from build123d import *

# Parameters (mm, degrees)
BOSS_EXTRUDE1_DEPTH = 50.8
FILLET1_R           = 2.032
FILLET2_R           = 1.27
SKETCH2_R           = 2.1971
SKETCH2_R_2         = 15.875
CUT_EXTRUDE1_DEPTH  = 104.011248837
SKETCH3_W           = 1.47561847
SKETCH3_H           = 5.061923893
CUT_EXTRUDE2_DEPTH  = 0.635


with BuildPart() as part:
    # Sketch1 → Boss-Extrude1 (new body)
    with BuildSketch(Plane.XY):
        Polygon((85.725, 0), (-85.725, 0), (-87.558087105, -3.175), (-54.56251922, -22.225), (-52.3875, -22.225), (-52.3875, -6.35), (52.3875, -6.35), (52.3875, -22.225), (54.56251922, -22.225), (87.558087105, -3.175), align=None)
    extrude(amount=BOSS_EXTRUDE1_DEPTH)

    # Fillet1
    fillet1_edges = [part.edges().sort_by_distance(p)[0] for p in [
        (-85.725, 0, 25.4),
        (85.725, 0, 25.4),
        (87.558087105, -3.175, 25.4),
        (52.3875, -6.35, 25.4),
        (-52.3875, -6.35, 25.4),
        (-87.558087105, -3.175, 25.4),
    ]]
    fillet(fillet1_edges, radius=FILLET1_R)

    # Fillet2
    fillet2_edges = [part.edges().sort_by_distance(p)[0] for p in [
        (54.56251922, -22.225, 25.4),
        (52.3875, -22.225, 25.4),
        (-52.3875, -22.225, 25.4),
        (-54.56251922, -22.225, 25.4),
    ]]
    fillet(fillet2_edges, radius=FILLET2_R)

    # Sketch2 → Cut-Extrude1 (cut, through all)
    with BuildSketch(Plane(origin=(0, 0, 0), x_dir=(1, 0, 0), z_dir=(0, 1, 0))):
        with Locations(Location((6.35, -35.56, 0), (0, 0, 180))):
            Circle(SKETCH2_R)
        with Locations(Location((-6.35, -35.56, 0), (0, 0, 180))):
            Circle(SKETCH2_R)
        with Locations(Location((-6.35, -15.24, 0), (0, 0, 180))):
            Circle(SKETCH2_R)
        with Locations(Location((6.35, -15.24, 0), (0, 0, 180))):
            Circle(SKETCH2_R)
        with Locations(Location((29.36875, -25.4, 0), (0, 0, 180))):
            Circle(SKETCH2_R_2)
        with Locations(Location((-29.36875, -25.4, 0), (0, 0, 180))):
            Circle(SKETCH2_R_2)
    extrude(amount=-CUT_EXTRUDE1_DEPTH, mode=Mode.SUBTRACT)

    # Sketch3 → Cut-Extrude2 (cut)
    with BuildSketch(Plane(origin=(0, 0, 0), x_dir=(1, 0, 0), z_dir=(0, 1, 0))):
        Polygon((61.952737106, -15.22945322), (63.428353296, -15.22945322), (63.428353296, -14.204150233), (66.787671186, -11.688640612), (69.723065901, -13.881379712), (69.723065901, -14.930594244), (71.198684372, -14.930594244), (71.198684372, -11.512394715), (69.723065901, -11.512394715), (69.723065901, -12.211960755), (67.929186974, -10.847171738), (69.723065901, -9.442854683), (69.723065901, -10.284273394), (71.198684372, -10.284273394), (71.198684372, -6.595230639), (69.723065901, -6.595230639), (69.723065901, -7.679269337), (66.787671186, -9.928245145), (63.428353296, -7.333914297), (63.428353296, -6.296371664), (61.952737106, -6.296371664), (61.952737106, -10.284273394), (63.428353296, -10.284273394), (63.428353296, -9.052344284), (65.662462767, -10.778941636), (63.428353296, -12.473735972), (63.428353296, -11.512394715), (61.952737106, -11.512394715), align=None)
        with Locations((65.679133813, -20.468824629)):
            Rectangle(SKETCH3_W, SKETCH3_H)
        with Locations((65.679133813, -30.181741323)):
            Rectangle(SKETCH3_W, SKETCH3_H)
        Polygon((64.586217495, -43.756476338), (66.339613015, -43.756476338), (69.106673825, -36.779987136), (67.706939797, -36.779987136), (65.470958353, -42.299591277), (63.202804515, -36.779987136), (61.803305338, -36.779987136), align=None)
    extrude(amount=-CUT_EXTRUDE2_DEPTH, mode=Mode.SUBTRACT)


solid = part.part
Build history of the part. All positions in model axes, mm. A direction names the side the tool comes from. Round coordinates to 2 decimals unless told otherwise and drop trailing zeros. Write each loop counter-clockwise with the first axis right and the second up, starting at its lowest first coordinate (ties: lowest second). Pieces come first, ordered by that corner, then holes. Notation, with made-up numbers: (37.25, -17) -> (77.25, -17) arc R24 cw to (77.25, 10) -> close; hole circle Ø7 at (73, 48.25). An arc over 180 degrees is marked (long way). Use one line per item in the form item = value.
Q1. Two-plate mould, pull along X, no slides. Class faces 4 (the flat face through (1, 0, 25)), 5 (the cylindrical face through (20.834, -3.131, 38.786)), 6 (the flat face through (-70.54, -13, 25.04)), 7 (the cylindrical face through (6.826, -3.131, 33.415)): released by +X, released by -X, zero draft, split by the parting line, or undercut.
Conclusion:
face_4 = zero draft
face_5 = undercut
face_6 = released by -X
face_7 = undercut
Q2. Drill centre lines: L1, parallel to Z at x = 6.35, y = -1.5; L2, parallel to X at y = -5.5, z = 18; L3, parallel to X at y = -5, z = 37.5. Where is each one in solid material? Low to high.
Conclusion:
L1 = 0 to 13.04, 17.44 to 33.36, 37.76 to 50.8
L2 = -83.53 to -43.41, -15.32 to 15.32, 43.41 to 83.53
L3 = -84.4 to -39.65, -19.09 to -7.38, -5.32 to 5.32, 7.38 to 19.09, 39.65 to 84.4
Q3. Drop flat-ended pins along their axis: P1, Ø7, axis at x = 6.35, z = 35.56, coming from the -Y side; P2, Ø4, axis at x = 66, y = -7.5, coming from the -Z side; P3, Ø0.7, axis at y = -0.5, z = 13.5, coming from the +X side; P4, Ø0.5, axis at y = -0.5, z = 14.5, coming from the -X side. Give the stop position or say it passes through.
Conclusion:
P1 = -6.35
P2 = 0
P3 = 86.2
P4 = -86.13
Q4. Band-saw the part on D-D, the plane x = 24.5. Write the cut outline in (y, z), then the cut area to 3 significant figures.
Conclusion:
outline = (-6.35, 0) -> (0, 0) -> (0, 10.29) -> (-6.35, 10.29) -> close; (-6.35, 40.51) -> (0, 40.51) -> (0, 50.8) -> (-6.35, 50.8) -> close
area = 131 mm²
Q5. Tool access for faces 1 (the flat face through (67.704, -0.313, 40.317)), 2 (the flat face through (52.388, -15, 25)), 3 (the cylindrical face through (-5.874, -3.131, 13.095)): list every direction of +Z, -Z, +X, -X, +Y, -Y with a clear straight run to the whole face (end or side of a thin tool).
Conclusion:
face_1 = +Y
face_2 = +Z, -Z, -Y
face_3 = +Y, -Y
Q6. Band-saw the part on B-B, the plane y = -12. Write the cut outline in (x, z), then the cut area to 3 significant figures.
Conclusion:
outline = (-72.27, 0) -> (-52.39, 0) -> (-52.39, 50.8) -> (-72.27, 50.8) -> close; (52.39, 0) -> (72.27, 0) -> (72.27, 50.8) -> (52.39, 50.8) -> close
area = 2,020 mm²
Q7. Band-saw the part on C-C, the plane z = 30.5. State how many separate pieces and enclosed holes the cut face has, then the cut area to 3 significant figures.
Conclusion:
separate_pieces = 3
enclosed_holes = 0
area = 1,210 mm²
Q8. Band-saw the part on A-A, the plane x = 6.35. Write the cut outline in (y, z).
Conclusion:
outline = (-6.35, 0) -> (0, 0) -> (0, 13.04) -> (-6.35, 13.04) -> close; (-6.35, 17.44) -> (0, 17.44) -> (0, 33.36) -> (-6.35, 33.36) -> close; (-6.35, 37.76) -> (0, 37.76) -> (0, 50.8) -> (-6.35, 50.8) -> close
